Geometry: final body of the model. Coordinates: model frame, mm. A direction names the side the tool comes from. Coordinates: 2 decimals unless noted, no trailing zeros. Order: outer loops, then holes, each group sorted by start corner. A loop starts at its lowest first (then second) coordinate and runs counter-clockwise, first axis right, second up. Notation, with made-up numbers: (-32, -5) -> (-17, -5) arc R24 cw to (-17, 9) -> close; hole circle Ø10 at (-25.5, 19). An arc over 180 degrees is marked (long way). Answer in a Markdown table with one row per item. Add a question column.
1) Set-up query: faces 1 (the face through (-1.61, 6.04, 2.76)), 2 (the face through (6.04, 1.61, 2.76)), 3 (the face through (-6.586, -2.65, 2.761)), 4 (the face through (-5.56, -4.37, 2.76)), 5 (the face through (-3.96, 6.836, 2.761)). Return all of +Z, -Z, +X, -X, +Y, -Y with unobstructed straight access to the full face (end or side cutting, diameter ignored); none if empty.
2) Section query A-A on x = 1.75. Return the cut outline in (y, z), then the cut area to 3 significant figures.
3) Contact query for a flat-ended pin moving along its axis: P1, Ø1.5, axis at x = -4.5, z = 3.5, coming from the -Y side. Output: stop coordinate, or through.
4) Section query B-B on x = -0.25. Return the cut outline in (y, z), then the cut area to 3 significant figures.
5) Section query C-C on y = -2.5. Return the cut outline in (x, z), then the cut area to 3 significant figures.
6) Section query D-D on x = 3.75. Return the cut outline in (y, z), then the cut area to 3 significant figures.
7) Pull-direction query (X, two-part tool) for faces 6 (the face through (-7.9, 0, 3)), 7 (the face through (0, 1.5, 3)), 8 (the face through (1.623, 6.035, 2.761)), 9 (the face through (3.94, 6.847, 2.761)); classes: +X half, -X half, draft (parallel to the pull), parting line (faces both ways), or undercut.
8) Ray query, line 1 (Y direction, x = 6.5, z = 4.9); line 2 (X direction, y = -7, z = 4.05); line 3 (X direction, y = -6.25, z = 2.45) (3 decimals). Return the intervals inside material, ascending. Write a range as from..to.
```python
from build123d import *

# Parameters (mm, degrees)
SKETCH1_R           = 6.25
BOSS_EXTRUDE1_DEPTH = 5.6
BOSS_EXTRUDE2_DEPTH = 5.6
CIRPATTERN1_COUNT   = 12
CUT_EXTRUDE1_DEPTH  = 7


with BuildPart() as part:
    # Sketch1 → Boss-Extrude1 (new body)
    with BuildSketch(Plane.XY):
        Circle(SKETCH1_R)
    extrude(amount=BOSS_EXTRUDE1_DEPTH)

    # Sketch3 → Boss-Extrude2 (add)
    with BuildSketch(Plane.XY):
        Polygon((-0.8, 7.9), (0.8, 7.9), (1.3, 5.7), (-1.3, 5.7), align=None)
    boss_extrude2 = extrude(amount=BOSS_EXTRUDE2_DEPTH)

    # CirPattern1: Boss-Extrude2 ×12 about axis
    cirpattern1_axis = Axis((0, 0, 0), (0, 0, 1))
    for i in range(1, CIRPATTERN1_COUNT):
        add(boss_extrude2.rotate(cirpattern1_axis, i * 360 / CIRPATTERN1_COUNT))

    # Sketch4 → Cut-Extrude1 (cut)
    with BuildSketch(Plane.XY):
        with BuildLine():
            Line((-2, -1.5), (2, -1.5))
            ThreePointArc((2, -1.5), (2.5, 0), (2, 1.5))
            Line((2, 1.5), (-2, 1.5))
            ThreePointArc((-2, 1.5), (-2.5, 0), (-2, -1.5))
        make_face()
    extrude(amount=CUT_EXTRUDE1_DEPTH, mode=Mode.SUBTRACT)


solid = part.part
```
Result:
| question | item | result |
|---|---|---|
| 1 | face 1 | +Z, -Z, +Y |
| 1 | face 2 | +Z, -Z, +X |
| 1 | face 3 | +Z, -Z, -X |
| 1 | face 4 | +Z, -Z, -Y |
| 1 | face 5 | +Z, -Z, -X, +Y |
| 2 | outline | (-6, 0) -> (-1.5, 0) -> (-1.5, 5.6) -> (-6, 5.6) -> close; (1.5, 0) -> (6, 0) -> (6, 5.6) -> (1.5, 5.6) -> close |
| 2 | area | 50.4 mm2 |
| 3 | P1 | y = -6.96 |
| 4 | outline | (-7.9, 0) -> (-1.5, 0) -> (-1.5, 5.6) -> (-7.9, 5.6) -> close; (1.5, 0) -> (7.9, 0) -> (7.9, 5.6) -> (1.5, 5.6) -> close |
| 4 | area | 71.7 mm2 |
| 5 | outline | (-6.42, 0) -> (6.42, 0) -> (6.42, 5.6) -> (-6.42, 5.6) -> close |
| 5 | area | 71.9 mm2 |
| 6 | outline | (-6.96, 0) -> (6.96, 0) -> (6.96, 5.6) -> (-6.96, 5.6) -> close |
| 6 | area | 77.9 mm2 |
| 7 | face 6 | -X half |
| 7 | face 7 | undercut |
| 7 | face 8 | undercut |
| 7 | face 9 | +X half |
| 8 | line 1 | -4.54..-2.57, -1.12..1.12, 2.57..4.54 |
| 8 | line 2 | -3.68..-3.03, -1..1, 3.03..3.68 |
| 8 | line 3 | -4.584..-2.339, -1.175..1.175, 2.339..4.584 |
